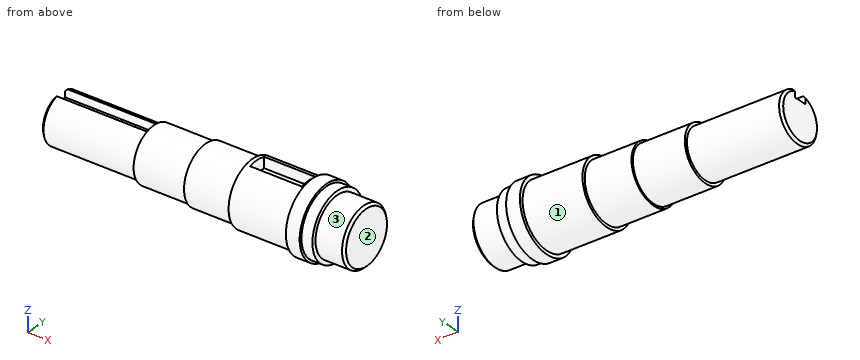
```python
from build123d import *

# Parameters (mm, degrees)
CUT_EXTRUDE_START   = 17.2
SKETCH_9_W          = 45
SKETCH_9_H          = 8
CUT_EXTRUDE_1_DEPTH = 36
CUT_EXTRUDE_START_2 = 13
SKETCH_12_W         = 81
SKETCH_12_H         = 6
CUT_EXTRUDE_4_DEPTH = 35
CHAMFER_1_SIZE      = 2


# Read off the part's stored shape, not the designer's step: 旋转3
with BuildPart() as part:
    # 旋转3 outline → 旋转3 (revolve)
    with BuildSketch(Plane(origin=(0, -27.284213334, 0), x_dir=(0, 1, 0), z_dir=(0, 0, -1))):
        Polygon((25, 155.634128986), (0, 155.634128986), (0, -110.465871014), (21, -110.465871014), (21, -28.465871014), (23.4, -28.465871014), (23.4, 16.534128986), (25, 16.534128986), (25, 57.134128986), (27.5, 57.134128986), (27.5, 109.134128986), (30.5, 109.134128986), (30.5, 121.134128986), (28.5, 121.134128986), (28.5, 130.634128986), (25, 130.634128986), align=None)
    revolve(axis=Axis((0, -27.284213334, 0), (1, 0, 0)))

    # 草图9 → 切除-拉伸1 (cut)
    with BuildSketch(Plane.XY.offset(CUT_EXTRUDE_START)):
        with Locations((83.134128986, -23.284213334)):
            Rectangle(SKETCH_9_W, SKETCH_9_H)
        with Locations((83.134128986, -31.284213334)):
            Rectangle(SKETCH_9_W, SKETCH_9_H)
    extrude(amount=CUT_EXTRUDE_1_DEPTH, mode=Mode.SUBTRACT)

    # 草图12 → 切除-拉伸4 (cut)
    with BuildSketch(Plane.XY.offset(CUT_EXTRUDE_START_2)):
        with Locations((-69.965871014, -24.284213334)):
            Rectangle(SKETCH_12_W, SKETCH_12_H)
        with Locations((-69.965871014, -30.284213334)):
            Rectangle(SKETCH_12_W, SKETCH_12_H)
    extrude(amount=CUT_EXTRUDE_4_DEPTH, mode=Mode.SUBTRACT)

    # 倒角1
    chamfer_1_edges = [part.edges().sort_by_distance(p)[0] for p in [
        (-110.465871014, -39.834113732, -16.837458241),
        (155.634128986, -52.284213334, 0),
    ]]
    chamfer(chamfer_1_edges, length=CHAMFER_1_SIZE)


solid = part.part
```
Work out the finished part from the listing and answer in its coordinate system (mm). Face numbers are marked on the shaded views. A direction names the side the tool comes from. Give positions to 0.01 mm unless a question says otherwise; leave off trailing zeros. Write each loop counter-clockwise with the first axis right and the second up, starting at its lowest first coordinate (ties: lowest second). Pieces come first, ordered by that corner, then holes. Notation, with made-up numbers: (-28.5, 61.5) -> (-15.5, 61.5) arc R4 cw to (-15.5, 68.5) -> close; hole circle Ø5 at (52.25, -30). An arc over 180 degrees is marked (long way). Write each question's results on one line, items separated by ' | '.
1. Find section D-D on x = 75. Determine the outline of the cut face in (y, z), and give its area (3 significant figures).
Data:
outline: (-35.28, 17.2) -> (-35.28, 26.31) arc R27.5 ccw (long way) to (-19.28, 26.31) -> (-19.28, 17.2) -> close | area: 2,220 mm^2
2. Find section C-C on x = 5.5. Determine the outline of the cut face in (y, z), and give its area (3 significant figures).
Data:
outline: circle Ø46.8 at (-27.28, 0) | area: 1,720 mm^2
3. Straight lines are drawn through the part: L1, parallel to X at y = -25.5, z = 16.5; L2, parallel to Y at x = -4.5, z = 1; L3, parallel to X at y = -48.5, z = 14. For each, find the intervals that lie inside material, in ascending order.
Data:
L1: -29.47 to 155.63 | L2: -50.66 to -3.91 | L3: 57.13 to 130.63
4. Each of these flat-tipped pins is pushed along its axis until it touches: pin 1 Ø3.5 at (x, z) = (-87.5, 16.5) entering from +Y; pin 2 Ø5 at (x, y) = (78, -29) entering from +Z; pin 3 Ø8 at (x, z) = (-76, 17.5) entering from -Y. Where does it stop, or does it pass through?
Data:
pin 1: y = -12.34 | pin 2: z = 17.2 | pin 3: y = -43.37
5. Find section B-B on x = -71. Determine the outline of the cut face in (y, z), and give its area (3 significant figures).
Data:
outline: (-33.28, 13) -> (-33.28, 20.12) arc R21 ccw (long way) to (-21.28, 20.12) -> (-21.28, 13) -> close | area: 1,290 mm^2
6. A tool of negligible diameter and unlimited length cuts with its end or side. For the marked faces 1, 2 and 3, from which of +Z, -Z, +X, -X, +Y, -Y can it reach the whole face along a straight path? Write none if from no direction.
Data:
face 1: -X | face 2: +Z, -Z, +X, +Y, -Y | face 3: +X
